Geometry: final body of the model. Coordinates: model frame, mm. A direction names the side the tool comes from. Give positions to 0.01 mm unless a question says otherwise; leave off trailing zeros. Loops run counter-clockwise (first coordinate to the right, second up) from the corner with the lowest first, then second, coordinate; pieces in that order, holes last. Notation, with made-up numbers: (-18.75, 83) -> (38.25, 83) arc R6 cw to (38.25, 94) -> close; hole circle Ø8 at (2, -24). An arc over 180 degrees is marked (long way). One line per question, with ' | ' between items. Start each with the question number.
Item 1: Section D-D on z = 24.5. Return loops of the section in (x, y).
Item 2: Pin query (flat end, axial travel): P1, Ø1.5, axis at y = -32, z = 55, coming from the +X side; P2, Ø1.5, axis at x = -16.5, z = 28, coming from the +Y side; P3, Ø8, axis at y = -16.5, z = 53.5, coming from the +X side; P4, Ø6, axis at x = -37, y = 19.5, coming from the -Z side. Return the tip coordinate at first contact, or that it passes through.
Item 3: Material intervals for line 1 along Z through (x, y) = (-18, 1); line 2 along Z through (x, y) = (14, 43); line 3 along Y through (x, z) = (0, 66.5), sorted ascending. Write a range as [from, to].
Item 4: Section C-C on z = 64.5. Return loops of the section in (x, y).
Item 5: Mould query, pull axis X, two halves, no side actions, for faces 3 (the flat face through (0, 0, 60)), 4 (the cylindrical face through (-29.97, 1.32, 65.07)), 5 (the flat face through (-1, 1, 0)), 6 (the flat face through (50, -1, 10)). Classes: released by +X, released by -X, zero draft, split by the parting line, or undercut.
Item 6: Set-up query: faces 1 (the flat face through (-45, 1, 20)), 2 (the flat face through (-1, 50, 10)). Return all of +Z, -Z, +X, -X, +Y, -Y with unobstructed straight access to the full face (end or side cutting, diameter ignored); none if empty.
Item 7: Section A-A on y = 0. Return loops of the section in (x, z).
from build123d import *

# Parameters (mm, degrees)
F0_W     = 100
F0_H     = 100
F1_DEPTH = 20
F2_R     = 42.5
F3_DEPTH = 50
F3_TAPER = 5
F4_R     = 30
F5_DEPTH = 10


with BuildPart() as f1:
    # F0 (on Top) → F1 (new body)
    with BuildSketch(Plane.XY):
        Rectangle(F0_W, F0_H)
    extrude(amount=F1_DEPTH)

    # F2 (on face) → F3 (join)
    with BuildSketch(Plane.XY.offset(20)):
        Circle(F2_R)
    extrude(amount=F3_DEPTH, taper=F3_TAPER)

    # F4 (on face) → F5 (cut)
    with BuildSketch(Plane.XY.offset(70)):
        Circle(F4_R)
    extrude(amount=-F5_DEPTH, mode=Mode.SUBTRACT)


solid = f1.part
Result sheet:
1) outline: circle Ø84.21 at (0, 0)
2) P1: stops at x = 24.06 | P2: stops at y = 38.73 | P3: stops at x = 37.59 | P4: stops at z = 0
3) line 1: z = [0, 60] | line 2: z = [0, 20] | line 3: y = [-38.43, -30], [30, 38.43]
4) outline: circle Ø77.21 at (0, 0); hole circle Ø60 at (0, 0)
5) face 3: undercut | face 4: undercut | face 5: zero draft | face 6: released by +X
6) face 1: +Z | face 2: +Z, -Z, +X, -X, +Y
7) outline: (-50, 0) -> (50, 0) -> (50, 20) -> (42.5, 20) -> (38.13, 70) -> (30, 70) -> (30, 60) -> (-30, 60) -> (-30, 70) -> (-38.13, 70) -> (-42.5, 20) -> (-50, 20) -> close
